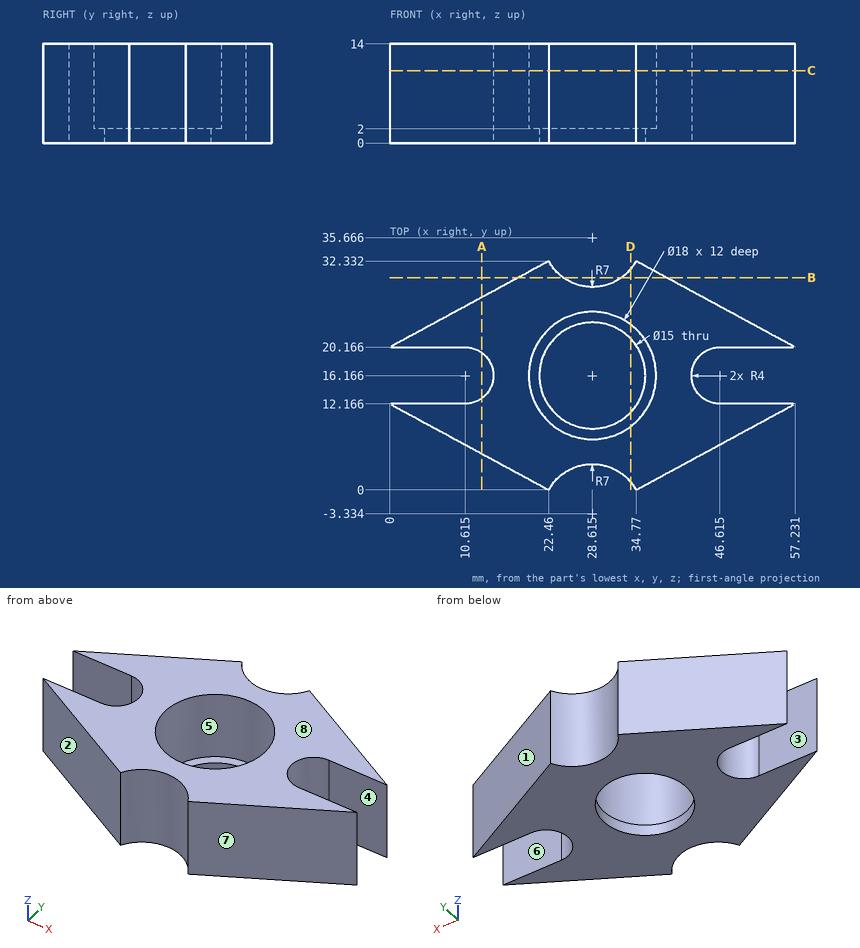
Job drawing, mm, ordinate dimensions from the low corner. One solid piece. A direction names the side the tool comes from. Give positions to 0.01 mm unless a question says otherwise; leave off trailing zeros. Loops run counter-clockwise (first coordinate to the right, second up) from the corner with the lowest first, then second, coordinate; pieces in that order, holes last.
Item 1: Slice it at A-A, the plane x = 13. List the corners of the cut face in (y, z) (1 decimal), and give its area (3 significant figures).
Answers follow:
outline: (5.1, 0) - (13, 0) - (13, 14) - (5.1, 14) - close; (19.4, 0) - (27.2, 0) - (27.2, 14) - (19.4, 14) - close
area: 219 mm2
Item 2: Flat gauge pins, fed straight in: pin 1 (1 mm diameter, centred on x = 9.5, z = 9.5, fed in from +Y); pin 2 (6 mm diameter, centred on x = 48.5, z = 2.5, fed in from +Y); pin 3 (3 mm diameter, centred on x = 50.5, z = 4, fed in from -Y). Where does each tip first touch, or does it go through?
Answers follow:
pin 1: stops at y = 25.58
pin 2: stops at y = 26.52
pin 3: stops at y = 7.71
Item 3: Drill centre lines: line 1 (X direction, y = 16.5, z = 9.25); line 2 (Y direction, x = 29, z = 6.5) (1 decimal); line 3 (Y direction, x = 51, z = 13.5) (1 decimal). Where is each one in solid material? Low to high.
Answers follow:
line 1: x = 14.6 to 19.62, 37.61 to 42.63
line 2: y = 3.7 to 7.2, 25.2 to 28.7
line 3: y = 8.8 to 12.2, 20.2 to 23.5
Item 4: Slice it at D-D, the plane x = 34. List the corners of the cut face in (y, z) (1 decimal).
Answers follow:
outline: (1.1, 0) - (10.9, 0) - (10.9, 2) - (9, 2) - (9, 14) - (1.1, 14) - close; (21.4, 0) - (31.2, 0) - (31.2, 14) - (23.4, 14) - (23.4, 2) - (21.4, 2) - close
Item 5: Pull direction Y, two halves, no side cores. Call the marked faces 6, 7 and 8: released by +Y, released by -Y, zero draft, split by the parting line, or undercut.
Answers follow:
face 6: undercut
face 7: released by -Y
face 8: zero draft
Item 6: Which spindle directions (+Z, -Z, +X, -X, +Y, -Y) get a long thin tool onto all of the face, cutting with end or side? Do the marked faces 1, 2, 3, 4 and 5. Say none if no direction does.
Answers follow:
face 1: +Z, -Z, +X, +Y
face 2: +Z, -Z, -X, -Y
face 3: +Z, -Z, -X
face 4: +Z, -Z, +X
face 5: +Z
Item 7: Slice it at C-C, the plane z = 10.25. List the corners of the cut face in (x, y) (1 decimal).
Answers follow:
outline: (0, 12.2) - (22.5, 0) arc R7 cw to (34.8, 0) - (57.2, 12.2) - (46.6, 12.2) arc R4 cw to (46.6, 20.2) - (57.2, 20.2) - (34.8, 32.3) arc R7 cw to (22.5, 32.3) - (0, 20.2) - (10.6, 20.2) arc R4 cw to (10.6, 12.2) - close; hole circle Ø18 at (28.6, 16.2)
Item 8: Slice it at B-B, the plane y = 30. List the corners of the cut face in (x, z) (1 decimal), and give its area (3 significant figures).
Answers follow:
outline: (18.2, 0) - (24.5, 0) - (24.5, 14) - (18.2, 14) - close; (32.7, 0) - (39.1, 0) - (39.1, 14) - (32.7, 14) - close
area: 178 mm2
